Build history of the part. All positions in model axes, mm. Coordinates: 2 decimals unless noted, no trailing zeros. Write each question's results on one line, items separated by ' | '. Start each with the question number.
Q1. Two-plate mould, pull along Y, no slides. Class faces 1 (the face through (-7.321, 23, 4)), 2 (the face through (141.254, 46.961, 3.802)), 3 (the face through (-5.895, -0.032, 3.802)): released by +Y, released by -Y, zero draft, split by the parting line, or undercut.
Q2. Drop a flat-ended pin along its axis: pin 1 Ø2 at (x, y) = (68, 39.5) entering from -Z. Give the stop position or say it passes through.
Q3. Drill centre lines: line 1 (Y direction, x = 0, z = 2.5); line 2 (X direction, y = 20, z = 1.75); line 3 (X direction, y = 45.5, z = 5). Where is each one in solid material? Low to high.
from build123d import *

# Parameters (mm, degrees)
F0_W     = 150
F0_H     = 50
F1_DEPTH = 7.5
F2_R     = 5
F3_R     = 5
F4_R     = 5
F5_R     = 5
F7_DEPTH = 25


with BuildPart() as f1:
    # F0 (on Top) → F1 (new body)
    with BuildSketch(Plane.XY):
        with Locations((67.679448, 23.464493)):
            Rectangle(F0_W, F0_H)
    extrude(amount=F1_DEPTH)

    # F2
    f2_edges = [f1.edges().sort_by_distance(p)[0] for p in [
        (-7.320552, -1.535507, 3.75),
    ]]
    fillet(f2_edges, radius=F2_R)

    # F3
    f3_edges = [f1.edges().sort_by_distance(p)[0] for p in [
        (-7.320552, 48.464493, 3.75),
    ]]
    fillet(f3_edges, radius=F3_R)

    # F4
    f4_edges = [f1.edges().sort_by_distance(p)[0] for p in [
        (142.679448, -1.535507, 3.75),
    ]]
    fillet(f4_edges, radius=F4_R)

    # F5
    f5_edges = [f1.edges().sort_by_distance(p)[0] for p in [
        (142.679448, 48.464493, 3.75),
    ]]
    fillet(f5_edges, radius=F5_R)

    # F6 (on face) → F7 (cut)
    with BuildSketch(Plane.XY.offset(7.5)):
        with BuildLine():
            ThreePointArc((0, 28.464493), (-3.535534, 19.928959), (5, 23.464493))
            ThreePointArc((5, 23.464493), (3.535534, 27.000027), (0, 28.464493))
        make_face()
    extrude(amount=-F7_DEPTH, mode=Mode.SUBTRACT)


solid = f1.part
Returned:
1) face 1: zero draft | face 2: released by +Y | face 3: released by -Y
2) pin 1: stops at z = 0
3) line 1: y = -1.54 to 18.46, 28.46 to 48.46 | line 2: x = -7.32 to -3.61, 3.61 to 142.68 | line 3: x = -6.89 to 142.25
